The model under review builds one solid part; all positions refer to its coordinate system, in mm. Face numbers are marked on the shaded views. A direction names the side the tool comes from. Round coordinates to 2 decimals unless told otherwise and drop trailing zeros. Order: outer loops, then holes, each group sorted by start corner. A loop starts at its lowest first (then second) coordinate and runs counter-clockwise, first axis right, second up.
```python
from build123d import *

# Parameters (mm, degrees)
F1_DEPTH       = 12
F2_DEPTH       = 8.5
F4_D           = 5
F4_CBORE_D     = 9.65
F4_CBORE_DEPTH = 3


with BuildPart() as f1:
    # F0 (on Front) → F1 (new body)
    with BuildSketch(Plane.XZ):
        Polygon((-10, 10), (-10, -7), (10, -7), (10, 10), (4.64, 10), (2.84, 8.2), (5.49934, 8.2), (5.49934, 6.56), (2.84, 3.90066), (-2.84, 3.90066), (-5.49934, 6.56), (-5.49934, 8.2), (-2.84, 8.2), (-4.64, 10), align=None)
        Polygon((4.64, 10), (-4.64, 10), (-2.84, 8.2), (-5.49934, 8.2), (-5.49934, 6.56), (-2.84, 3.90066), (2.84, 3.90066), (5.49934, 6.56), (5.49934, 8.2), (2.84, 8.2), align=None)
    extrude(amount=F1_DEPTH)

    # F0 (on Front) → F2 (cut)
    with BuildSketch(Plane.XZ):
        Polygon((4.64, 10), (-4.64, 10), (-2.84, 8.2), (-5.49934, 8.2), (-5.49934, 6.56), (-2.84, 3.90066), (2.84, 3.90066), (5.49934, 6.56), (5.49934, 8.2), (2.84, 8.2), align=None)
    extrude(amount=F2_DEPTH, mode=Mode.SUBTRACT)

    # F4 (through all)
    with Locations(Plane.XZ.offset(12)):
        with Locations((0, 0)):
            CounterBoreHole(F4_D / 2, F4_CBORE_D / 2, F4_CBORE_DEPTH)


solid = f1.part
```
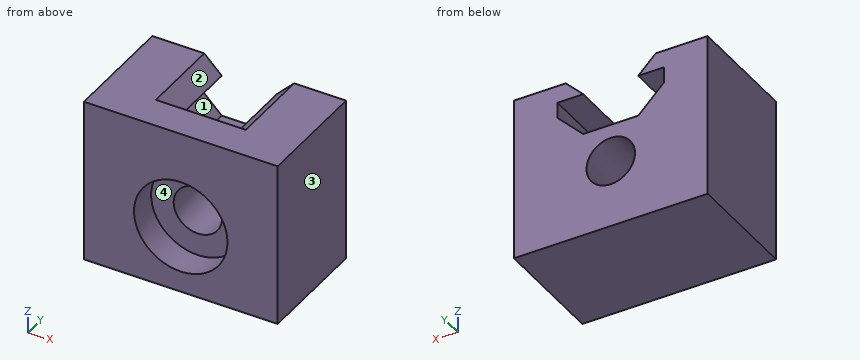
(1) Insertion check: pin 1 (3 mm diameter, centred on x = 1, z = 4, fed in from -Y); pin 2 (6 mm diameter, centred on x = 1, y = -4, fed in from +Z); pin 3 (1.8 mm diameter, centred on x = 2.5, z = 6.5, fed in from +Y). Each pin has a flat end and moves straight along its axis. Give the tip position at first contact, or say it passes through.
Data:
pin 1: stops at y = -12
pin 2: stops at z = 9.36
pin 3: stops at y = -8.5
(2) Consider section D-D (z = 7.75). Write out the cut boundary in (x, y), and give its area (3 significant figures).
Data:
outline: (-10, -12) - (10, -12) - (10, 0) - (5.5, 0) - (5.5, -8.5) - (-5.5, -8.5) - (-5.5, 0) - (-10, 0) - close
area: 147 mm2
(3) Consider section A-A (z = 0). Write out the cut boundary in (x, y) (3 decimals).
Data:
outline: (-10, -12) - (-4.825, -12) - (-4.825, -9) - (-2.5, -9) - (-2.5, 0) - (-10, 0) - close; (2.5, -9) - (4.825, -9) - (4.825, -12) - (10, -12) - (10, 0) - (2.5, 0) - close
(4) To check wall thickness, follow probe 1 along Z at (x, y) = (0, -2.75); probe 2 along Z at (x, y) = (0, -9.9) (3 decimals); probe 3 along X at (y, z) = (-6.5, 7). State the ranges of each line that lie inside material, in increasing order.
Data:
probe 1: z = -7 to -2.5, 2.5 to 3.9
probe 2: z = -7 to -4.825, 4.825 to 10
probe 3: x = -10 to -5.5, 5.5 to 10
(5) Consider section C-C (y = -1). Write out the cut boundary in (x, z).
Data:
outline: (-10, -7) - (10, -7) - (10, 10) - (4.64, 10) - (2.84, 8.2) - (5.5, 8.2) - (5.5, 6.56) - (2.84, 3.9) - (-2.84, 3.9) - (-5.5, 6.56) - (-5.5, 8.2) - (-2.84, 8.2) - (-4.64, 10) - (-10, 10) - close; hole circle Ø5 at (0, 0)
(6) For the marked faces 1, 2, 3 and 4, list the 3-axis set-ups (+Z, -Z, +X, -X, +Y, -Y) from which the entire face can be reached by the end or side of a thin tool; tool diameter is ignored.
Data:
face 1: +Y
face 2: +Z, +Y
face 3: +Z, -Z, +X, +Y, -Y
face 4: -Y
(7) Consider section B-B (x = 0). Write out the cut boundary in (y, z) (3 decimals).
Data:
outline: (-12, -7) - (0, -7) - (0, -2.5) - (-9, -2.5) - (-9, -4.825) - (-12, -4.825) - close; (-12, 4.825) - (-9, 4.825) - (-9, 2.5) - (0, 2.5) - (0, 3.901) - (-8.5, 3.901) - (-8.5, 10) - (-12, 10) - close
